Autodesk Fusion 360 part; units mm, degrees
sketch "Sketch1" plane through (0, 0, 0) normal (0, 0, 1) x (1, 0, 0)
  line L0 (0, 0) -> (50, 0)
  line L1 (50, 0) -> (50, 50)
  line L2 (50, 50) -> (0, 50)
  line L3 (0, 50) -> (0, 0)
  circle A0 centre (25, 25) radius 4.5
  dimension "d1" = 50
  dimension "d2" = 50
  dimension "d3" = 9
  dimension "d4" = 25
  dimension "d5" = 25
extrude "Extrude1" add sketch "Sketch1" along normal blind 5
Verification items for the finished model (mm, model axes). Give positions to 0.01 mm unless a question says otherwise; leave off trailing zeros. Order: outer loops, then holes, each group sorted by start corner. A loop starts at its lowest first (then second) coordinate and runs counter-clockwise, first axis right, second up. Notation, with made-up numbers: (56.25, -0.5) -> (96.25, -0.5) arc R23 ccw to (96.25, 18.5) -> close; hole circle Ø3 at (77, 40.25). An arc over 180 degrees is marked (long way). Answer as CSV lines item,"result".
Q1. Release check for a two-part mould opening along Y. For faces 1 (the cylindrical face through (21.68, 21.96, 2.46)), 2 (the flat face through (0, 25, 2)), 3 (the flat face through (25, 0, 2)), 4 (the flat face through (25, 50, 2)) record: +Y half, -Y half, draft (parallel to the pull), parting line (faces both ways), or undercut.
Solutions:
face 1,"undercut"
face 2,"draft"
face 3,"-Y half"
face 4,"+Y half"
Q2. Sectioned sample at B-B on z = 3.65. Record the cut outline in (x, y), plus the area to 3 significant figures.
Solutions:
outline,"(0, 0) -> (50, 0) -> (50, 50) -> (0, 50) -> close; hole circle Ø9 at (25, 25)"
area,"2,440 mm²"
Q3. Scan lines: probe 1 along Y at (x, z) = (25, 2.8); probe 2 along X at (y, z) = (28, 4.25); probe 3 along X at (y, z) = (22.5, 2.55). Record each from-to range of solid material in increasing order.
Solutions:
probe 1,"y = 0 to 20.5, 29.5 to 50"
probe 2,"x = 0 to 21.65, 28.35 to 50"
probe 3,"x = 0 to 21.26, 28.74 to 50"
Q4. Depth check by flat-ended pin: pin 1 (1.5 mm diameter, centred on x = 14, z = 1.5, fed in from -Y). Enter the tip coordinate at first touch or a pass-through.
Solutions:
pin 1,"stops at y = 0"
Q5. Sectioned sample at A-A on x = 25. Record the cut outline in (y, z).
Solutions:
outline,"(0, 0) -> (20.5, 0) -> (20.5, 5) -> (0, 5) -> close; (29.5, 0) -> (50, 0) -> (50, 5) -> (29.5, 5) -> close"
